from build123d import *

# Parameters (mm, degrees)
SKETCH2_R           = 1.25
SKETCH2_R_2         = 1.75
SKETCH2_R_3         = 2.75
BOSS_EXTRUDE1_DEPTH = 2


with BuildPart() as part:
    # Sketch2 → Boss-Extrude1 (new body)
    with BuildSketch(Plane(origin=(0, 0, 0), x_dir=(1, 0, 0), z_dir=(0, 1, 0))):
        with BuildLine():
            Line((24.142135624, -6.273144482), (24.142135624, 0))
            Line((24.142135624, 0), (24.142135624, 6.273144482))
            ThreePointArc((24.142135624, 6.273144482), (24.827649201, 9.717819404), (26.779731412, 12.637594949))
            Line((26.779731412, 12.637594949), (56.468368159, 42.304675289))
            ThreePointArc((56.468368159, 42.304675289), (63.53883973, 45.231039727), (70.608156448, 42.301886572))
            Line((70.608156448, 42.301886572), (75.694551302, 37.21517354))
            ThreePointArc((75.694551302, 37.21517354), (78.858485001, 33.634695425), (80, 28.994949366))
            ThreePointArc((80, 28.994949366), (87.5, 21.494949366), (95, 28.994949366))
            Line((95, 28.994949366), (95, 35.208152802))
            ThreePointArc((95, 35.208152802), (94.238795325, 39.034987125), (92.071067812, 42.279220614))
            Line((92.071067812, 42.279220614), (42.279220614, 92.071067812))
            ThreePointArc((42.279220614, 92.071067812), (39.034987125, 94.238795325), (35.208152802, 95))
            Line((35.208152802, 95), (-35.208152802, 95))
            ThreePointArc((-35.208152802, 95), (-39.034987125, 94.238795325), (-42.279220614, 92.071067812))
            Line((-42.279220614, 92.071067812), (-92.071067812, 42.279220614))
            ThreePointArc((-92.071067812, 42.279220614), (-94.238795325, 39.034987125), (-95, 35.208152802))
            Line((-95, 35.208152802), (-95, 28.994949366))
            ThreePointArc((-95, 28.994949366), (-87.5, 21.494949366), (-80, 28.994949366))
            ThreePointArc((-80, 28.994949366), (-79.238795325, 32.82178369), (-77.071067812, 36.066017178))
            Line((-77.071067812, 36.066017178), (-70.710678119, 42.426406871))
            ThreePointArc((-70.710678119, 42.426406871), (-63.639610307, 45.355339059), (-56.568542495, 42.426406871))
            Line((-56.568542495, 42.426406871), (-26.777420433, 12.63528481))
            ThreePointArc((-26.777420433, 12.63528481), (-24.827023831, 9.716310016), (-24.142135624, 6.273144482))
            Line((-24.142135624, 6.273144482), (-24.142135624, -6.273144482))
            ThreePointArc((-24.142135624, -6.273144482), (-24.827023831, -9.716310016), (-26.777420433, -12.63528481))
            Line((-26.777420433, -12.63528481), (-56.568542495, -42.426406871))
            ThreePointArc((-56.568542495, -42.426406871), (-63.639766689, -45.355339058), (-70.710899273, -42.42618571))
            Line((-70.710899273, -42.42618571), (-77.018051571, -36.11863887))
            ThreePointArc((-77.018051571, -36.11863887), (-79.224438078, -32.856262892), (-80, -28.994949366))
            ThreePointArc((-80, -28.994949366), (-87.518972201, -21.532505276), (-95, -29.032987782))
            Line((-95, -29.032987782), (-95, -35.208152802))
            ThreePointArc((-95, -35.208152802), (-94.238795325, -39.034987125), (-92.071067812, -42.279220614))
            Line((-92.071067812, -42.279220614), (-42.279220614, -92.071067812))
            ThreePointArc((-42.279220614, -92.071067812), (-39.034987125, -94.238795325), (-35.208152802, -95))
            Line((-35.208152802, -95), (35.208152802, -95))
            ThreePointArc((35.208152802, -95), (39.034987125, -94.238795325), (42.279220614, -92.071067812))
            Line((42.279220614, -92.071067812), (92.071067812, -42.279220614))
            ThreePointArc((92.071067812, -42.279220614), (94.238795325, -39.034987125), (95, -35.208152802))
            Line((95, -35.208152802), (95, -28.994949366))
            ThreePointArc((95, -28.994949366), (87.5, -21.494949366), (80, -28.994949366))
            ThreePointArc((80, -28.994949366), (79.238795325, -32.82178369), (77.071067812, -36.066017178))
            Line((77.071067812, -36.066017178), (70.710678119, -42.426406871))
            ThreePointArc((70.710678119, -42.426406871), (63.639610307, -45.355339059), (56.568542495, -42.426406871))
            Line((56.568542495, -42.426406871), (26.777420433, -12.63528481))
            ThreePointArc((26.777420433, -12.63528481), (24.827023831, -9.716310016), (24.142135624, -6.273144482))
        make_face()
        with Locations(Location((-61.871843354, -61.871843354, 0), (0, 0, 270))):
            Circle(SKETCH2_R, mode=Mode.SUBTRACT)
        with Locations(Location((-35.928385408, -86.738795325, 0), (0, 0, 270))):
            Circle(SKETCH2_R_2, mode=Mode.SUBTRACT)
        with BuildLine():
            Line((-36.066017178, -77.071067812), (-42.49385989, -70.643225099))
            ThreePointArc((-42.49385989, -70.643225099), (-45.422791224, -63.568024355), (-42.488012626, -56.495247042))
            Line((-42.488012626, -56.495247042), (-40.972308908, -54.982133019))
            ThreePointArc((-40.972308908, -54.982133019), (-37.730173876, -52.818813648), (-33.90728957, -52.059244135))
            Line((-33.90728957, -52.059244135), (-28.020223739, -52.059244135))
            ThreePointArc((-28.020223739, -52.059244135), (-23.037212382, -49.995213249), (-20.973181496, -45.012201892))
            Line((-20.973181496, -45.012201892), (-20.973181496, -39.298846649))
            ThreePointArc((-20.973181496, -39.298846649), (-20.205038234, -35.45530386), (-18.018617262, -32.20223937))
            Line((-18.018617262, -32.20223937), (-12.595254252, -26.81798261))
            ThreePointArc((-12.595254252, -26.81798261), (-9.664285168, -24.842115466), (-6.198377489, -24.147770665))
            Line((-6.198377489, -24.147770665), (6.198377489, -24.147770665))
            ThreePointArc((6.198377489, -24.147770665), (9.664285168, -24.842115466), (12.595254252, -26.81798261))
            Line((12.595254252, -26.81798261), (18.018617262, -32.20223937))
            ThreePointArc((18.018617262, -32.20223937), (20.205038234, -35.45530386), (20.973181496, -39.298846649))
            Line((20.973181496, -39.298846649), (20.973181496, -45.012201892))
            ThreePointArc((20.973181496, -45.012201892), (23.037212382, -49.995213249), (28.020223739, -52.059244135))
            Line((28.020223739, -52.059244135), (33.90728957, -52.059244135))
            ThreePointArc((33.90728957, -52.059244135), (37.730173876, -52.818813648), (40.972308908, -54.982133019))
            Line((40.972308908, -54.982133019), (42.488012626, -56.495247042))
            ThreePointArc((42.488012626, -56.495247042), (45.309602969, -63.534055428), (42.380741747, -70.528908358))
            Line((42.380741747, -70.528908358), (37.216069936, -75.693257115))
            ThreePointArc((37.216069936, -75.693257115), (33.63539271, -78.858119754), (28.994949366, -80))
            Line((28.994949366, -80), (-28.994949366, -80))
            ThreePointArc((-28.994949366, -80), (-32.82178369, -79.238795325), (-36.066017178, -77.071067812))
        make_face(mode=Mode.SUBTRACT)
        with Locations(Location((-28.020223739, -45.012201892, 0), (0, 0, 270))):
            Circle(SKETCH2_R_3, mode=Mode.SUBTRACT)
        with Locations(Location((-86.738795325, -35.928385408, 0), (0, 0, 270))):
            Circle(SKETCH2_R_2, mode=Mode.SUBTRACT)
        with Locations(Location((-28, -28, 0), (0, 0, 270))):
            Circle(SKETCH2_R, mode=Mode.SUBTRACT)
        with BuildLine():
            ThreePointArc((0, 15.25), (10.783378413, 10.783378413), (15.25, 0))
            ThreePointArc((15.25, 0), (-10.783378413, -10.783378413), (0, 15.25))
        make_face(mode=Mode.SUBTRACT)
        with Locations(Location((35.928385408, -86.738795325, 0), (0, 0, 270))):
            Circle(SKETCH2_R_2, mode=Mode.SUBTRACT)
        with Locations(Location((28.020223739, -45.012201892, 0), (0, 0, 270))):
            Circle(SKETCH2_R_3, mode=Mode.SUBTRACT)
        with Locations(Location((61.871843354, -61.871843354, 0), (0, 0, 270))):
            Circle(SKETCH2_R, mode=Mode.SUBTRACT)
        with Locations(Location((28, -28, 0), (0, 0, 270))):
            Circle(SKETCH2_R, mode=Mode.SUBTRACT)
        with Locations(Location((86.738795325, -35.928385408, 0), (0, 0, 270))):
            Circle(SKETCH2_R_2, mode=Mode.SUBTRACT)
        with Locations(Location((-86.738795325, 35.928385408, 0), (0, 0, 270))):
            Circle(SKETCH2_R_2, mode=Mode.SUBTRACT)
        with Locations(Location((-28, 28, 0), (0, 0, 270))):
            Circle(SKETCH2_R, mode=Mode.SUBTRACT)
        with Locations(Location((-61.871843354, 61.871843354, 0), (0, 0, 270))):
            Circle(SKETCH2_R, mode=Mode.SUBTRACT)
        with Locations(Location((-28.020223739, 45.012201892, 0), (0, 0, 270))):
            Circle(SKETCH2_R_3, mode=Mode.SUBTRACT)
        with BuildLine():
            Line((6.206060109, 24.155528451), (0, 24.155528451))
            Line((0, 24.155528451), (-6.206060109, 24.155528451))
            ThreePointArc((-6.206060109, 24.155528451), (-9.666929362, 24.847771886), (-12.595254252, 26.81798261))
            Line((-12.595254252, 26.81798261), (-18.018617262, 32.20223937))
            ThreePointArc((-18.018617262, 32.20223937), (-20.205038234, 35.45530386), (-20.973181496, 39.298846649))
            Line((-20.973181496, 39.298846649), (-20.973181496, 45.012201892))
            ThreePointArc((-20.973181496, 45.012201892), (-23.037212382, 49.995213249), (-28.020223739, 52.059244135))
            Line((-28.020223739, 52.059244135), (-33.90728957, 52.059244135))
            ThreePointArc((-33.90728957, 52.059244135), (-37.730173876, 52.818813648), (-40.972308908, 54.982133019))
            Line((-40.972308908, 54.982133019), (-42.488012626, 56.495247042))
            ThreePointArc((-42.488012626, 56.495247042), (-45.422992439, 63.568239451), (-42.493839938, 70.643647124))
            Line((-42.493839938, 70.643647124), (-36.065796017, 77.071288966))
            ThreePointArc((-36.065796017, 77.071288966), (-32.821639211, 79.238855169), (-28.994949366, 80))
            Line((-28.994949366, 80), (28.994949366, 80))
            ThreePointArc((28.994949366, 80), (32.82178369, 79.238795325), (36.066017178, 77.071067812))
            Line((36.066017178, 77.071067812), (42.49385989, 70.643225099))
            ThreePointArc((42.49385989, 70.643225099), (45.422791224, 63.568024355), (42.488012626, 56.495247042))
            Line((42.488012626, 56.495247042), (40.972308908, 54.982133019))
            ThreePointArc((40.972308908, 54.982133019), (37.730173876, 52.818813648), (33.90728957, 52.059244135))
            Line((33.90728957, 52.059244135), (28.020223739, 52.059244135))
            ThreePointArc((28.020223739, 52.059244135), (23.037212382, 49.995213249), (20.973181496, 45.012201892))
            Line((20.973181496, 45.012201892), (20.973181496, 39.298846649))
            ThreePointArc((20.973181496, 39.298846649), (20.205038234, 35.45530386), (18.018617262, 32.20223937))
            Line((18.018617262, 32.20223937), (12.595254252, 26.81798261))
            ThreePointArc((12.595254252, 26.81798261), (9.666929362, 24.847771886), (6.206060109, 24.155528451))
        make_face(mode=Mode.SUBTRACT)
        with Locations(Location((-35.928385408, 86.738795325, 0), (0, 0, 270))):
            Circle(SKETCH2_R_2, mode=Mode.SUBTRACT)
        with Locations(Location((28, 28, 0), (0, 0, 270))):
            Circle(SKETCH2_R, mode=Mode.SUBTRACT)
        with Locations(Location((86.738795325, 35.928385408, 0), (0, 0, 270))):
            Circle(SKETCH2_R_2, mode=Mode.SUBTRACT)
        with Locations(Location((28.020223739, 45.012201892, 0), (0, 0, 270))):
            Circle(SKETCH2_R_3, mode=Mode.SUBTRACT)
        with Locations(Location((35.928385408, 86.738795325, 0), (0, 0, 270))):
            Circle(SKETCH2_R_2, mode=Mode.SUBTRACT)
        with Locations(Location((61.871843354, 61.871843354, 0), (0, 0, 270))):
            Circle(SKETCH2_R, mode=Mode.SUBTRACT)
    extrude(amount=BOSS_EXTRUDE1_DEPTH)


solid = part.part
Work out the finished part from the listing and answer in its coordinate system (mm). Round coordinates to 2 decimals unless told otherwise and drop trailing zeros. Use one line per item in the form item = value.
(1) Find section A-A on y = 1.3. Give the number of separate pieces and of enclosed holes in the cut face, then the cut area to 3 significant figures.
Answer list:
separate_pieces = 1
enclosed_holes = 23
area = 13,500 mm2
(2) Straight lines are drawn through the part: line 1 (Z direction, x = -18, y = 1.2); line 2 (X direction, y = 0.6, z = -26); line 3 (Z direction, x = -1, y = 1.15). For each, find the intervals that lie inside material, in ascending order.
Answer list:
line_1 = -95 to -80, -32.18 to 32.18, 80 to 95
line_2 = -94.38 to -80.62, -40.14 to -11.66, 11.66 to 40.15, 80.62 to 94.38
line_3 = -95 to -80, -24.16 to -15.22, 15.22 to 24.15, 80 to 95
(3) For a pull along X with two mould halves and no side action, classify faces 1 (the flat face through (67.52, 0.99, -66.83)), 2 (the flat face through (-67.52, 0.99, 66.83)), 3 (the flat face through (-73.935, 0.986, -39.202)) as released by +X, released by -X, zero draft, split by the parting line, or undercut.
Answer list:
face_1 = released by +X
face_2 = released by -X
face_3 = undercut
(4) Flat-ended cylindrical pins translate along their axes: P1, Ø18.5, axis at x = 0, z = 0, coming from the -Y side; P2, Ø1, axis at y = 1.5, z = 1.5, coming from the -X side; P3, Ø1, axis at y = 0.5, z = -41, coming from the +X side. Find the tip coordinate at first contact, or state that the pin passes through.
Answer list:
P1 = through
P2 = -24.14
P3 = 93.49
